Model file for the job. Use its own axes, mm. A direction names the side the tool comes from. Round coordinates to 2 decimals unless told otherwise and drop trailing zeros. Write each loop counter-clockwise with the first axis right and the second up, starting at its lowest first coordinate (ties: lowest second). Pieces come first, ordered by that corner, then holes. Notation, with made-up numbers: (48.5, 32.25) - (81.5, 32.25) arc R13 ccw to (81.5, 43.25) - close; hole circle Ø5 at (75, 76.5). An arc over 180 degrees is marked (long way). Answer as a JSON object with one key per item and string values. Group by question number.
from build123d import *

# Parameters (mm, degrees)
SKETCH1_R           = 1.825
BOSS_EXTRUDE1_DEPTH = 1.98
SKETCH2_R           = 0.945
BOSS_EXTRUDE2_DEPTH = 20
CUT_EXTRUDE1_DEPTH  = 1
CHAMFER1_SIZE       = 0.2


with BuildPart() as part:
    # Sketch1 → Boss-Extrude1 (new body)
    with BuildSketch(Plane(origin=(0, 0, 0), x_dir=(1, 0, 0), z_dir=(0, 1, 0))):
        Circle(SKETCH1_R)
    extrude(amount=BOSS_EXTRUDE1_DEPTH)

    # Sketch2 → Boss-Extrude2 (add)
    with BuildSketch(Plane(origin=(0, 1.98, 0), x_dir=(1, 0, 0), z_dir=(0, 1, 0))):
        Circle(SKETCH2_R)
    extrude(amount=BOSS_EXTRUDE2_DEPTH)

    # Sketch3 → Cut-Extrude1 (cut)
    with BuildSketch(Plane.XZ):
        Polygon((0.458993464, -0.795), (0.917986928, 0), (0.458993464, 0.795), (-0.458993464, 0.795), (-0.917986928, 0), (-0.458993464, -0.795), align=None)
    extrude(amount=-CUT_EXTRUDE1_DEPTH, mode=Mode.SUBTRACT)

    # Chamfer1
    chamfer1_edges = [part.edges().sort_by_distance(p)[0] for p in [
        (-0.945, 21.98, 0),
    ]]
    chamfer(chamfer1_edges, length=CHAMFER1_SIZE)


solid = part.part
(1) Slice it at A-A (x = 0). Write the cut outline in (y, z) (3 decimals), then the cut area to 3 significant figures.
(2) Slice it at B-B (y = 17.5). Write the cut outline in (x, z) (3 decimals), then the cut area to 3 significant figures.
(3) Drill centre lines: line 1 (X direction, y = 4, z = 0) (3 decimals); line 2 (Y direction, x = 1, z = 1.2); line 3 (Z direction, x = -0.1, y = 20.25). Where is each one in solid material? Low to high. Write a range as from..to.
(4) 3-axis set-ups, long thin cutter, end or side, ignore diameter. For faces 1 (the cylindrical face through (1.74, 0.98, -0.55)), 2 (the flat face through (0, 0.5, -0.795)): which of +Z, -Z, +X, -X, +Y, -Y reach the whole face in a straight line?
(5) Slice it at C-C (z = 1.55). Write the cut outline in (x, y), then the cut area to 3 significant figures.
(6) Flat gauge pins, fed straight in: pin 1 (1.5 mm diameter, centred on x = -1, y = 19.5, fed in from -Z); pin 2 (1.5 mm diameter, centred on y = 8.5, z = -1, fed in from +X); pin 3 (1.8 mm diameter, centred on x = -1, z = -1, fed in from +Y); pin 4 (1 mm diameter, centred on x = -1, y = 15, fed in from -Z). Where does each tip first touch, or does it go through?
(7) Pull direction Z, two halves, no side cores. Call faces 3 (the flat face through (1, 1.98, 1)), 4 (the cylindrical face through (-0.205, 11.741, 0.923)), 5 (the flat face through (0, 1, 0)): pulls with the +Z half, pulls with the -Z half, needs draft (parallel to the pull), parting line crosses it, or undercut.
Answer:
{
 "1": {"outline": "(0, -1.825) - (1.98, -1.825) - (1.98, -0.945) - (21.78, -0.945) - (21.98, -0.745) - (21.98, 0.745) - (21.78, 0.945) - (1.98, 0.945) - (1.98, 1.825) - (0, 1.825) - (0, 0.795) - (1, 0.795) - (1, -0.795) - (0, -0.795) - close", "area": "43.4 mm²"},
 "2": {"outline": "circle Ø1.89 at (0, 0)", "area": "2.81 mm²"},
 "3": {"line 1": "-0.945..0.945", "line 2": "0..1.98", "line 3": "-0.94..0.94"},
 "4": {"face 1": "+Y, -Y", "face 2": "-Y"},
 "5": {"outline": "(-0.96, 0) - (0.96, 0) - (0.96, 1.98) - (-0.96, 1.98) - close", "area": "3.82 mm²"},
 "6": {"pin 1": "z = -0.91", "pin 2": "x = 0.91", "pin 3": "y = 21.98", "pin 4": "z = -0.8"},
 "7": {"face 3": "needs draft", "face 4": "parting line crosses it", "face 5": "undercut"}
}
